Geometry check sheet. Reference: the model listing, model coordinates, mm. A direction names the side the tool comes from. Round coordinates to 2 decimals unless told otherwise and drop trailing zeros. Loops run counter-clockwise (first coordinate to the right, second up) from the corner with the lowest first, then second, coordinate; pieces in that order, holes last. Notation, with made-up numbers: (-38.5, 42.25) -> (-9.5, 42.25) arc R31 cw to (-9.5, 67.25) -> close; hole circle Ø10 at (67, -10). An arc over 180 degrees is marked (long way). Use a Markdown table: item, result. Add a question column.
Q1. Material ranges on L1, parallel to X at y = -0.6, z = -2.6; L2, parallel to X at y = -1.4, z = 1.2; L3, parallel to Z at x = 3.25, y = 0.65, recorded low to high.
Q2. Gauge pin test, flat ends, axial feed: P1, Ø1, axis at x = 3, z = -1, coming from the +Y side; P2, Ø0.8, axis at y = -1, z = -2.5, coming from the -X side; P3, Ø1, axis at x = 3.5, y = -2, coming from the -Z side. Record the tip position at first contact, or that the pin passes through.
Q3. Sectioned sample at D-D, the plane y = 0.7. Enter the section's corners in (x, z), then the cut area to 3 significant figures.
Q4. Release check for a two-part mould opening along X. For faces 3 (the face through (0.26, 1.16, 0.04)), 4 (the face through (7.62, 0, 0)), 5 (the face through (4, 0, -2.159)) record: released by +X, released by -X, zero draft, split by the parting line, or undercut.
Q5. Sectioned sample at C-C, the plane x = 4.5. Enter the section's corners in (y, z).
Q6. Sectioned sample at A-A, the plane y = -0.55. Enter the section's corners in (x, z).
Q7. Sectioned sample at B-B, the plane z = 0. Enter the section's corners in (x, y).
Q8. Set-up check for faces 1 (the face through (3.76, 0.13, 2.92)), 2 (the face through (0.309, -1, 0)): record each of +Z, -Z, +X, -X, +Y, -Y from which the full face is reachable in a straight line by a thin tool's end or side.
```python
from build123d import *

# Parameters (mm, degrees)
SKETCH3_R                      = 2.921
BOSS_EXTRUDE2_DEPTH            = 7.62
CUT_EXTRUDE1_REACH             = 4.921
CUT_EXTRUDE1_DIRECTION_2_REACH = 4.921
CUT_EXTRUDE2_REACH             = 4.921
SKETCH5_W                      = 1.524
SKETCH5_H                      = 0.762
CUT_EXTRUDE2_DIRECTION_2_REACH = 4.921


with BuildPart() as part:
    # Sketch3 → Boss-Extrude2 (new body)
    with BuildSketch(Plane(origin=(0, 0, 0), x_dir=(0, 0, -1), z_dir=(1, 0, 0))):
        Circle(SKETCH3_R)
    extrude(amount=BOSS_EXTRUDE2_DEPTH)

    # Sketch4 → Cut-Extrude1 (cut, up to next)
    with BuildSketch(Plane.XY, mode=Mode.PRIVATE) as cut_extrude1_sk1:
        with BuildLine():
            Line((0.308789988, 0), (0.308789988, -2.921))
            Line((0.308789988, -2.921), (0, -2.921))
            Line((0, -2.921), (0, 2.921))
            ThreePointArc((0, 2.921), (0.231378009, 1.468638167), (0.308789988, 0))
        make_face()
    cut_extrude1_tool1 = extrude(cut_extrude1_sk1.sketch, amount=-CUT_EXTRUDE1_REACH, mode=Mode.PRIVATE) & part.part
    add(cut_extrude1_tool1.solids().sort_by_distance((0.142074, -0.436129, 0))[0], mode=Mode.SUBTRACT)

    # Sketch4 → Cut-Extrude1 direction 2 (cut, up to next)
    with BuildSketch(Plane.XY, mode=Mode.PRIVATE) as cut_extrude1_direction_2_sk1:
        with BuildLine():
            Line((0.308789988, 0), (0.308789988, -2.921))
            Line((0.308789988, -2.921), (0, -2.921))
            Line((0, -2.921), (0, 2.921))
            ThreePointArc((0, 2.921), (0.231378009, 1.468638167), (0.308789988, 0))
        make_face()
    cut_extrude1_direction_2_tool1 = extrude(cut_extrude1_direction_2_sk1.sketch, amount=CUT_EXTRUDE1_DIRECTION_2_REACH, mode=Mode.PRIVATE) & part.part
    add(cut_extrude1_direction_2_tool1.solids().sort_by_distance((0.142074, -0.436129, 0))[0], mode=Mode.SUBTRACT)

    # Sketch5 → Cut-Extrude2 (cut, up to next)
    with BuildSketch(Plane(origin=(0, 0, 0), x_dir=(1, 0, 0), z_dir=(0, 1, 0)), mode=Mode.PRIVATE) as cut_extrude2_sk1:
        with Locations((3.610789988, 2.54)):
            Rectangle(SKETCH5_W, SKETCH5_H)
    cut_extrude2_tool1 = extrude(cut_extrude2_sk1.sketch, amount=-CUT_EXTRUDE2_REACH, mode=Mode.PRIVATE) & part.part
    add(cut_extrude2_tool1.solids().sort_by_distance((3.61079, 0, -2.54))[0], mode=Mode.SUBTRACT)

    # Sketch5 → Cut-Extrude2 direction 2 (cut, up to next)
    with BuildSketch(Plane(origin=(0, 0, 0), x_dir=(1, 0, 0), z_dir=(0, 1, 0)), mode=Mode.PRIVATE) as cut_extrude2_direction_2_sk1:
        with Locations((3.610789988, 2.54)):
            Rectangle(SKETCH5_W, SKETCH5_H)
    cut_extrude2_direction_2_tool1 = extrude(cut_extrude2_direction_2_sk1.sketch, amount=CUT_EXTRUDE2_DIRECTION_2_REACH, mode=Mode.PRIVATE) & part.part
    add(cut_extrude2_direction_2_tool1.solids().sort_by_distance((3.61079, 0, -2.54))[0], mode=Mode.SUBTRACT)


solid = part.part
```
Values:
| question | item | result |
|---|---|---|
| 1 | L1 | 0.31 to 2.85, 4.37 to 7.62 |
| 1 | L2 | 0.31 to 7.62 |
| 1 | L3 | -2.16 to 2.85 |
| 2 | P1 | y = 2.88 |
| 2 | P2 | x = 0.31 |
| 2 | P3 | z = -2.16 |
| 3 | outline | (0.29, -2.84) -> (2.85, -2.84) -> (2.85, -2.16) -> (4.37, -2.16) -> (4.37, -2.84) -> (7.62, -2.84) -> (7.62, 2.84) -> (0.29, 2.84) -> close |
| 3 | area | 40.5 mm^2 |
| 4 | face 3 | released by -X |
| 4 | face 4 | released by +X |
| 4 | face 5 | undercut |
| 5 | outline | circle Ø5.84 at (0, 0) |
| 6 | outline | (0.31, -2.87) -> (2.85, -2.87) -> (2.85, -2.16) -> (4.37, -2.16) -> (4.37, -2.87) -> (7.62, -2.87) -> (7.62, 2.87) -> (0.31, 2.87) -> close |
| 7 | outline | (0, 2.92) arc R13.97 cw to (0.31, 0) -> (0.31, -2.92) -> (7.62, -2.92) -> (7.62, 2.92) -> close |
| 8 | face 1 | +X, -X |
| 8 | face 2 | +Z, -Z, -X, -Y |
